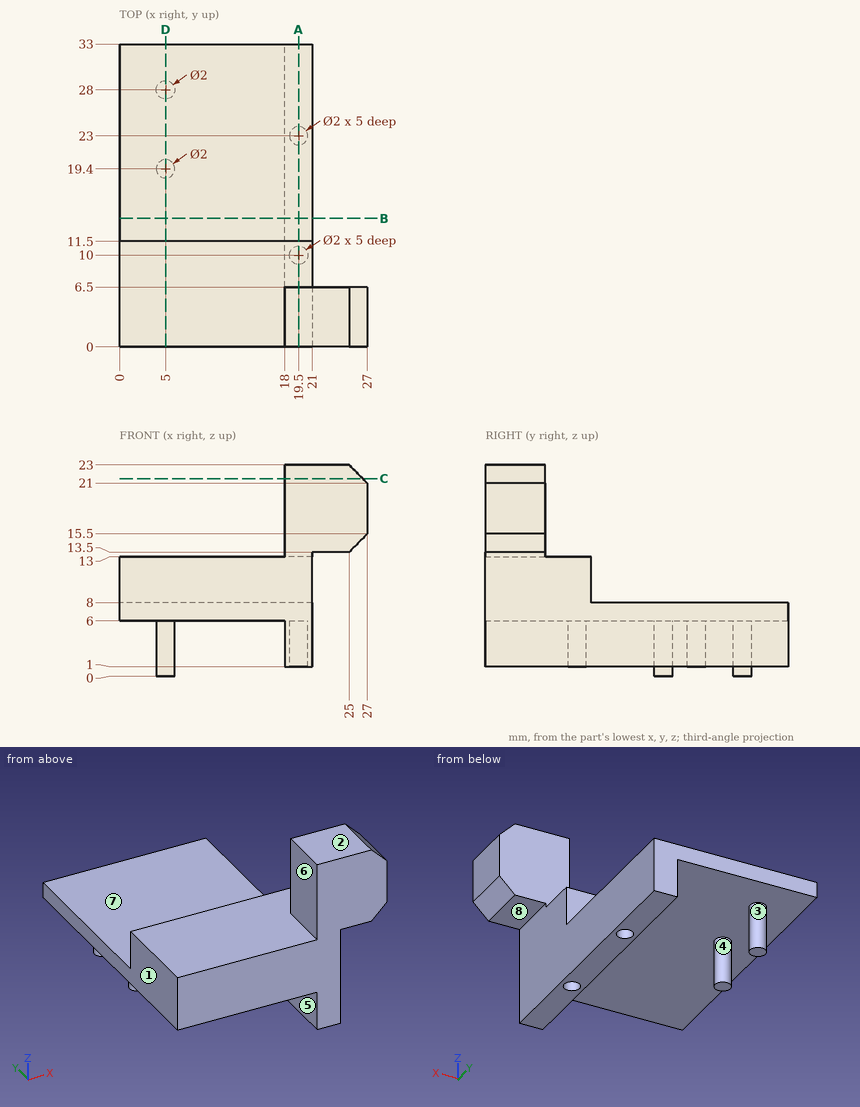
Geometry check sheet. Reference: drawing and pictorial views, mm from the part's lowest x, y, z. A direction names the side the tool comes from. Round coordinates to 2 decimals unless told otherwise and drop trailing zeros. Loops run counter-clockwise (first coordinate to the right, second up) from the corner with the lowest first, then second, coordinate; pieces in that order, holes last. Notation, with made-up numbers: (12, 86) - (27, 86) arc R17 cw to (27, 104) - close; hole circle Ø2 at (-28.5, 73). An arc over 180 degrees is marked (long way). Use a Markdown table: item, result. Add a question column.
1. Release check for a two-part mould opening along X. For the marked faces 1, 2 and 3 record: released by +X, released by -X, zero draft, split by the parting line, or undercut.
2. Section check B-B, the plane y = 14. Record the boundary of the cut face in (x, z), plus the area to 3 significant figures.
3. Section check A-A, the plane x = 19.5. Record the boundary of the cut face in (y, z), plus the area to 4 significant figures.
4. Section check C-C, the plane z = 21.5. Record the boundary of the cut face in (x, y), plus the area to 4 significant figures.
5. Access from +Z, -Z, +X, -X, +Y, -Y to the whole of each face (thin tool, end or side, straight path). Record for the marked faces 4, 5, 6, 7 and 8.
6. Thickness scan on probe 1 along Y at (x, z) = (19.5, 4.9); probe 2 along Z at (x, y) = (9, 17); probe 3 along X at (y, z) = (10, 4.35). Record the ranges inside material, lowest first. Write a range as [from, to].
7. Gauge pin test, flat ends, axial feed: pin 1 (1.2 mm diameter, centred on x = 19.5, y = 23, fed in from +Z); pin 2 (4.5 mm diameter, centred on x = 21.5, z = 18.5, fed in from +Y); pin 3 (2 mm diameter, centred on x = 14, y = 22, fed in from -Z). Record the tip position at first contact, or that the pin passes through.
8. Section check D-D, the plane x = 5. Record the boundary of the cut face in (y, z).
Checks:
| question | item | result |
|---|---|---|
| 1 | face 1 | released by -X |
| 1 | face 2 | zero draft |
| 1 | face 3 | undercut |
| 2 | outline | (0, 6) - (18, 6) - (18, 1) - (21, 1) - (21, 8) - (0, 8) - close |
| 2 | area | 57.0 mm^2 |
| 3 | outline | (0, 1) - (9, 1) - (9, 6) - (11, 6) - (11, 1) - (22, 1) - (22, 6) - (24, 6) - (24, 1) - (33, 1) - (33, 8) - (11.5, 8) - (11.5, 13) - (6.5, 13) - (6.5, 23) - (0, 23) - close |
| 3 | area | 333.5 mm^2 |
| 4 | outline | (18, 0) - (26.5, 0) - (26.5, 6.5) - (18, 6.5) - close |
| 4 | area | 55.25 mm^2 |
| 5 | face 4 | -Z |
| 5 | face 5 | -Z, +Y, -Y |
| 5 | face 6 | +Z, -X, +Y, -Y |
| 5 | face 7 | +Z, +X, -X, +Y |
| 5 | face 8 | -Z, +X, +Y, -Y |
| 6 | probe 1 | y = [0, 9], [11, 22], [24, 33] |
| 6 | probe 2 | z = [6, 8] |
| 6 | probe 3 | x = [18, 18.5], [20.5, 21] |
| 7 | pin 1 | stops at z = 8 |
| 7 | pin 2 | stops at y = 6.5 |
| 7 | pin 3 | stops at z = 6 |
| 8 | outline | (0, 6) - (18.4, 6) - (18.4, 0) - (20.4, 0) - (20.4, 6) - (27, 6) - (27, 0) - (29, 0) - (29, 6) - (33, 6) - (33, 8) - (11.5, 8) - (11.5, 13) - (0, 13) - close |
